```python
from build123d import *

# Parameters (mm, degrees)
F1_DEPTH = 19.05
F3_DEPTH = 1225.55
F4_W     = 19.05
F4_H     = 38.1
F5_DEPTH = 25.4
F6_W     = 63.5
F6_H     = 19.05
F7_DEPTH = 19.05


with BuildPart() as f1:
    # F0 (on Top) → F1 (new body)
    with BuildSketch(Plane.XY):
        Polygon((-16.216737, -254), (-270.216737, 0), (-270.216737, -254), align=None)
        Polygon((-16.216737, -254), (-270.216737, -254), (-270.216737, -508), (237.783263, -508), align=None)
        Polygon((237.783263, -508), (-270.216737, -508), (-270.216737, -762), (491.783263, -762), align=None)
    extrude(amount=F1_DEPTH)

    # F2 (on face) → F3 (join)
    with BuildSketch(Plane.XY.offset(19.05)):
        with BuildLine():
            ThreePointArc((-206.716737, -508), (-219.416737, -495.3), (-232.116737, -508))
            Line((-232.116737, -508), (-206.716737, -508))
        make_face()
        with BuildLine():
            ThreePointArc((199.683263, -508), (186.983263, -495.3), (174.283263, -508))
            Line((174.283263, -508), (199.683263, -508))
        make_face()
        with BuildLine():
            Line((199.683263, -508), (174.283263, -508))
            ThreePointArc((174.283263, -508), (186.983263, -520.7), (199.683263, -508))
        make_face()
        with BuildLine():
            ThreePointArc((148.883263, -508), (136.183263, -495.3), (123.483263, -508))
            Line((123.483263, -508), (148.883263, -508))
        make_face()
        with BuildLine():
            Line((148.883263, -508), (123.483263, -508))
            ThreePointArc((123.483263, -508), (136.183263, -520.7), (148.883263, -508))
        make_face()
        with BuildLine():
            ThreePointArc((98.083263, -508), (85.383263, -495.3), (72.683263, -508))
            Line((72.683263, -508), (98.083263, -508))
        make_face()
        with BuildLine():
            Line((98.083263, -508), (72.683263, -508))
            ThreePointArc((72.683263, -508), (85.383263, -520.7), (98.083263, -508))
        make_face()
        with BuildLine():
            ThreePointArc((47.283263, -508), (34.583263, -495.3), (21.883263, -508))
            Line((21.883263, -508), (47.283263, -508))
        make_face()
        with BuildLine():
            Line((47.283263, -508), (21.883263, -508))
            ThreePointArc((21.883263, -508), (34.583263, -520.7), (47.283263, -508))
        make_face()
        with BuildLine():
            ThreePointArc((-3.516737, -508), (-16.216737, -495.3), (-28.916737, -508))
            Line((-28.916737, -508), (-3.516737, -508))
        make_face()
        with BuildLine():
            Line((-3.516737, -508), (-28.916737, -508))
            ThreePointArc((-28.916737, -508), (-16.216737, -520.7), (-3.516737, -508))
        make_face()
        with BuildLine():
            ThreePointArc((-54.316737, -508), (-67.016737, -495.3), (-79.716737, -508))
            Line((-79.716737, -508), (-54.316737, -508))
        make_face()
        with BuildLine():
            Line((-54.316737, -508), (-79.716737, -508))
            ThreePointArc((-79.716737, -508), (-67.016737, -520.7), (-54.316737, -508))
        make_face()
        with BuildLine():
            ThreePointArc((-105.116737, -508), (-117.816737, -495.3), (-130.516737, -508))
            Line((-130.516737, -508), (-105.116737, -508))
        make_face()
        with BuildLine():
            Line((-105.116737, -508), (-130.516737, -508))
            ThreePointArc((-130.516737, -508), (-117.816737, -520.7), (-105.116737, -508))
        make_face()
        with BuildLine():
            ThreePointArc((-155.916737, -508), (-168.616737, -495.3), (-181.316737, -508))
            Line((-181.316737, -508), (-155.916737, -508))
        make_face()
        with BuildLine():
            Line((-155.916737, -508), (-181.316737, -508))
            ThreePointArc((-181.316737, -508), (-168.616737, -520.7), (-155.916737, -508))
        make_face()
        with BuildLine():
            Line((-206.716737, -508), (-232.116737, -508))
            ThreePointArc((-232.116737, -508), (-219.416737, -520.7), (-206.716737, -508))
        make_face()
        with BuildLine():
            ThreePointArc((-194.016737, -254), (-206.716737, -241.3), (-219.416737, -254))
            Line((-219.416737, -254), (-194.016737, -254))
        make_face()
        with BuildLine():
            ThreePointArc((-67.016737, -254), (-79.716737, -241.3), (-92.416737, -254))
            Line((-92.416737, -254), (-67.016737, -254))
        make_face()
        with BuildLine():
            Line((-67.016737, -254), (-92.416737, -254))
            ThreePointArc((-92.416737, -254), (-79.716737, -266.7), (-67.016737, -254))
        make_face()
        with BuildLine():
            ThreePointArc((-130.516737, -254), (-143.216737, -241.3), (-155.916737, -254))
            Line((-155.916737, -254), (-130.516737, -254))
        make_face()
        with BuildLine():
            Line((-130.516737, -254), (-155.916737, -254))
            ThreePointArc((-155.916737, -254), (-143.216737, -266.7), (-130.516737, -254))
        make_face()
        with BuildLine():
            Line((-194.016737, -254), (-219.416737, -254))
            ThreePointArc((-219.416737, -254), (-206.716737, -266.7), (-194.016737, -254))
        make_face()
    extrude(amount=F3_DEPTH)

    # F4 (on face) → F5 (cut)
    with BuildSketch(Plane.XY):
        with Locations((-235.291737, -565.15)):
            Rectangle(F4_W, F4_H)
        with Locations((-235.291737, -666.75)):
            Rectangle(F4_W, F4_H)
        with Locations((253.658263, -565.15)):
            Rectangle(F4_W, F4_H)
        with Locations((253.658263, -666.75)):
            Rectangle(F4_W, F4_H)
    extrude(amount=F5_DEPTH, mode=Mode.SUBTRACT)

    # F6 (on face) → F7 (join)
    with BuildSketch(Plane(origin=(-270.216737, 0, 0), x_dir=(0, -1, 0), z_dir=(-1, 0, 0))):
        with Locations((552.45, 9.525)):
            Rectangle(F6_W, F6_H)
        with Locations((692.15, 9.525)):
            Rectangle(F6_W, F6_H)
        with Locations((69.85, 9.525)):
            Rectangle(F6_W, F6_H)
        with Locations((209.55, 9.525)):
            Rectangle(F6_W, F6_H)
    extrude(amount=F7_DEPTH)


solid = f1.part
```
Source: CAD feature listing. Evaluate the final solid. Frame: model axes, mm. A direction names the side the tool comes from. Give positions to 0.01 mm unless a question says otherwise; leave off trailing zeros. Loops run counter-clockwise (first coordinate to the right, second up) from the corner with the lowest first, then second, coordinate; pieces in that order, holes last. Notation, with made-up numbers: (-17.5, -38.5) - (28.5, -38.5) arc R31 cw to (28.5, -3.5) - close; hole circle Ø2 at (23, 38.25). An arc over 180 degrees is marked (long way). Use CSV: the item, a comma, the result in double quotes.
1) Pin query (flat end, axial travel): P1, Ø21, axis at y = -26, z = 8, coming from the -X side; P2, Ø21, axis at x = -276, z = 10, coming from the -Y side; P3, Ø10, axis at y = -513, z = 466, coming from the +X side; P4, Ø9.5, axis at y = -570.5, z = 11, coming from the +X side. Return the tip coordinate at first contact, or that it passes through.
Worked out:
P1,"stops at x = -270.22"
P2,"stops at y = -762"
P3,"stops at x = 199.68"
P4,"stops at x = 305.03"
2) Cut plane A-A (z = 791). Count the separate pieces of the cut face and the enclosed holes in it, and give its area (3 significant figures).
Worked out:
separate pieces,"12"
enclosed holes,"0"
area,"6,080 mm^2"
3) Cut plane B-B (x = 289.5). Output: boundary loops of the cut face in (y, z).
Worked out:
outline,"(-762, 0) - (-559.72, 0) - (-559.72, 19.05) - (-762, 19.05) - close"
4) Cut plane C-C (y = -161.5). Output: boundary loops of the cut face in (x, z).
Worked out:
outline,"(-270.22, 0) - (-108.72, 0) - (-108.72, 19.05) - (-270.22, 19.05) - close"
5) Set-up query: faces 4 (the cylindrical face through (-150.04, -264.71, 623.25)), 5 (the flat face through (-169, -508, 1244.6)). Return all of +Z, -Z, +X, -X, +Y, -Y with unobstructed straight access to the full face (end or side cutting, diameter ignored); none if empty.
Worked out:
face 4,"+Z"
face 5,"+Z, +X, -X, +Y, -Y"
6) Line query: line 1 (Z direction, x = -119.5, y = -461); line 2 (Y direction, x = -119.5, z = 374.5); line 3 (Y direction, x = -56, z = 350). Output: solid intervals per line, ascending.
Worked out:
line 1,"z = 0 to 19.05"
line 2,"y = -520.59 to -495.41"
line 3,"y = -514.32 to -501.68"
7) Mould query, pull axis Y, two halves, no side actions, for faces 1 (the cylindrical face through (-65.36, -520.59, 623.25)), 2 (the flat face through (-207, -254, 1244.6)), 3 (the cylindrical face through (-14.56, -520.59, 623.25)). Classes: +Y half, -Y half, draft (parallel to the pull), parting line (faces both ways), or undercut.
Worked out:
face 1,"undercut"
face 2,"draft"
face 3,"parting line"
